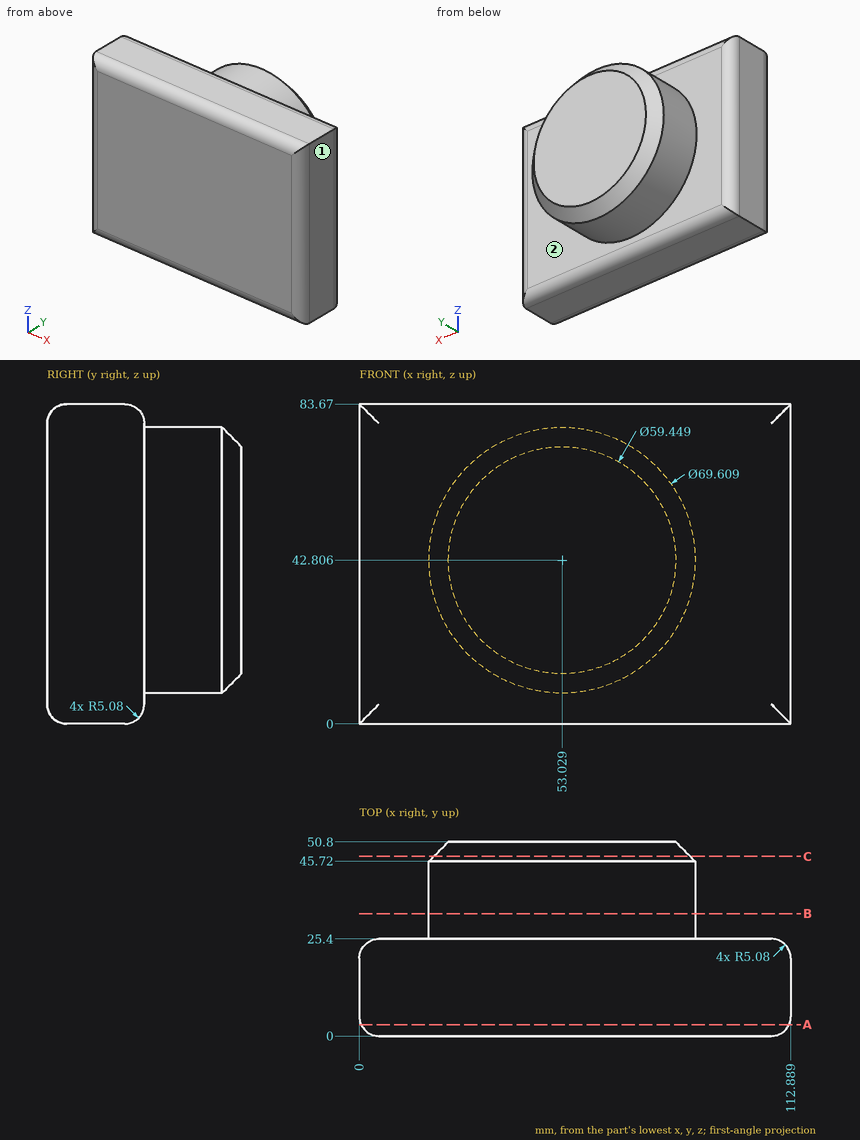
Job drawing, mm, ordinate dimensions from the low corner. One solid piece. A direction names the side the tool comes from. Coordinates: 2 decimals unless noted, no trailing zeros. Write each loop counter-clockwise with the first axis right and the second up, starting at its lowest first coordinate (ties: lowest second). Pieces come first, ordered by that corner, then holes. Notation, with made-up numbers: (65, -21) -> (89, -21) arc R15 cw to (89, 1) -> close; hole circle Ø9 at (-12, 71.25). An arc over 180 degrees is marked (long way). Use CSV: the item, a comma, the result in double quotes. Start each with the question number.
Item 1: Band-saw the part on C-C, the plane y = 47. Write the cut outline in (x, z) (1 decimal).
Item 2: Tool access for the marked faces 1 and 2: list every direction of +Z, -Z, +X, -X, +Y, -Y with a clear straight run to the whole face (end or side of a thin tool).
Item 3: Wall check: probe 1 along Y at (x, z) = (10.5, 51.5); probe 2 along X at (y, z) = (21, 45) (1 decimal); probe 3 along X at (y, z) = (30, 41). Give the ranges that are in metal, low to high.
Item 4: Band-saw the part on A-A, the plane y = 3. Write the cut outline in (x, z) (1 decimal).
Item 5: Drop flat-ended pins along their axis: P1, Ø5, axis at y = 39, z = 22.5, coming from the -X side (1 decimal); P2, Ø6, axis at x = 68, y = 33, coming from the +Z side; P3, Ø8, axis at x = 18.5, z = 65, coming from the +Y side. Give the stop position or say it passes through.
Item 6: Band-saw the part on B-B, the plane y = 32. Write the cut outline in (x, z) (1 decimal), plus the area to 3 significant figures.
Response values:
1,outline,"circle Ø67 at (53, 42.8)"
2,face 1,"+Z, -Z, +X, +Y, -Y"
2,face 2,"+Y"
3,probe 1,"y = 0 to 25.4"
3,probe 2,"x = 0 to 112.8"
3,probe 3,"x = 18.27 to 87.79"
4,outline,"(0.4, 0.4) -> (112.4, 0.4) -> (112.4, 83.2) -> (0.4, 83.2) -> close"
5,P1,"stops at x = 23.1"
5,P2,"stops at z = 75.49"
5,P3,"stops at y = 25.4"
6,outline,"circle Ø69.6 at (53, 42.8)"
6,area,"3,810 mm2"
